from build123d import *

# Parameters (mm, degrees)
SKETCH_1_R          = 22.5
EXTRUDE_1_DEPTH     = 95
SKETCH_2_W          = 1
SKETCH_2_H          = 1
FILLET_1_R          = 2
SKETCH_3_R          = 5
EXTRUDE_2_DEPTH     = 2
SKETCH_4_R          = 3
CUT_EXTRUDE_1_DEPTH = 1


with BuildPart() as part:
    # Эскиз1 → Бобышка-Вытянуть1 (new body)
    with BuildSketch(Plane(origin=(0, 0, 0), x_dir=(1, 0, 0), z_dir=(0, 1, 0))):
        with Locations(Location((0, 0, 0), (0, 0, 270))):
            Circle(SKETCH_1_R)
    extrude(amount=EXTRUDE_1_DEPTH)

    # Эскиз2 → Вырез-Повернуть1 (revolve, cut)
    with BuildSketch(Plane.XY, mode=Mode.PRIVATE) as cut_revolve_1_sk:
        with Locations((22, 84.5)):
            Rectangle(SKETCH_2_W, SKETCH_2_H)
    revolve(cut_revolve_1_sk.sketch.rotate(Axis((0, 95, 0), (0, -1, 0)), 180), axis=Axis((0, 95, 0), (0, -1, 0)), mode=Mode.SUBTRACT)

    # Скругление1
    fillet_1_edges = [part.edges().sort_by_distance(p)[0] for p in [
        (0, 95, -22.5),
    ]]
    fillet(fillet_1_edges, radius=FILLET_1_R)

    # Эскиз3 → Бобышка-Вытянуть2 (add)
    with BuildSketch(Plane(origin=(0, 95, 0), x_dir=(1, 0, 0), z_dir=(0, 1, 0))):
        with Locations(Location((0, 0, 0), (0, 0, 270))):
            Circle(SKETCH_3_R)
    extrude(amount=EXTRUDE_2_DEPTH)

    # Эскиз4 → Вырез-Вытянуть1 (cut)
    with BuildSketch(Plane(origin=(0, 97, 0), x_dir=(1, 0, 0), z_dir=(0, 1, 0))):
        with Locations(Location((0, 0, 0), (0, 0, 270))):
            Circle(SKETCH_4_R)
    extrude(amount=-CUT_EXTRUDE_1_DEPTH, mode=Mode.SUBTRACT)


solid = part.part
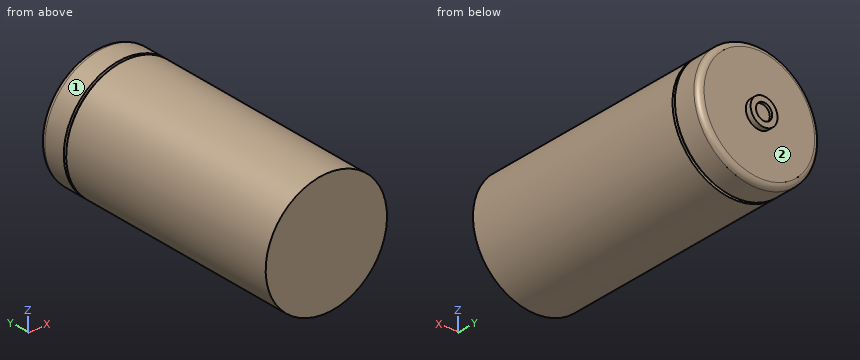
Can you work these out from the model? Positions are in its coordinate system, mm. Face numbers are marked on the shaded views. A direction names the side the tool comes from. Coordinates: 2 decimals unless noted, no trailing zeros. Write each loop counter-clockwise with the first axis right and the second up, starting at its lowest first coordinate (ties: lowest second). Pieces come first, ordered by that corner, then holes. Notation, with made-up numbers: (15.5, 62.5) -> (48.5, 62.5) arc R16 ccw to (48.5, 71.5) -> close; hole circle Ø8 at (66, 66). An arc over 180 degrees is marked (long way). Answer as CSV lines item,"result".
1) If I drill on line 1 (X direction, y = 96.45, z = 0); line 2 (Y direction, x = -12, z = 14.5); line 3 (Y direction, x = 19.5, z = 10), over which ranges is the centre line in solid material (lowest first)? Write a range as from..to.
Check result:
line 1,"-5..-3, 3..5"
line 2,"0..95"
line 3,"0..84, 85..94.41"
2) Will these pins go through, and if not, where does the flat tip stop? P1, Ø3, axis at y = 65.5, z = 1.5, coming from the +X side; P2, Ø2, axis at x = -9, y = 73, coming from the -Z side; P3, Ø8, axis at y = 33, z = 16, coming from the -X side.
Check result:
P1,"x = 22.5"
P2,"z = -21.03"
P3,"x = -19.03"
3) If we section it at B-B on y = 43: Please give me the cut outline in (x, z), then the cut area to 3 significant figures.
Check result:
outline,"circle Ø45 at (0, 0)"
area,"1,590 mm²"
4) On a 3-axis mill with a long thin cutter (end or side, diameter ignored), from which of +Z, -Z, +X, -X, +Y, -Y can I reach the whole of each face in a straight line? I mean the marked faces 1 and 2. Say none if no direction works.
Check result:
face 1,"+Y, -Y"
face 2,"+Y"
5) If we section it at A-A on z = 0: Please give me the cut outline in (x, y), then the cut area to 3 significant figures.
Check result:
outline,"(-22.5, 0) -> (22.5, 0) -> (22.5, 84) -> (21.5, 84) -> (21.5, 85) -> (22.5, 85) -> (22.5, 93) arc R2 ccw to (20.5, 95) -> (5, 95) -> (5, 97) -> (3, 97) -> (3, 96) -> (-3, 96) -> (-3, 97) -> (-5, 97) -> (-5, 95) -> (-20.5, 95) arc R2 ccw to (-22.5, 93) -> (-22.5, 85) -> (-21.5, 85) -> (-21.5, 84) -> (-22.5, 84) -> close"
area,"4,290 mm²"
